Autodesk Inventor part; units mm, degrees
ref_plane "YZ Plane" through (0, 0, 0) normal (1, 0, 0) x (0, 1, 0)
ref_plane "XZ Plane" through (0, 0, 0) normal (0, 1, 0) x (-1, 0, 0)
ref_plane "XY Plane" through (0, 0, 0) normal (0, 0, 1) x (1, 0, 0)
sketch "Sketch1" plane through (0, 0, 0) normal (0, 0, 1) x (1, 0, 0)
  circle A0 centre (0, 0) radius 1.5
  circle A1 centre (0, 0) radius 3
  line L0 (0, 3) -> (28, 3)
  line L1 (28, 3) -> (28, -3)
  line L2 (28, -3) -> (0, -3)
  line L3 (0, -3) -> (0, 3)
  line L4 (28, 3) -> (10, 3)
  line L5 (10, 3) -> (10, 59)
  line L6 (10, 59) -> (28, 59)
  line L7 (28, 59) -> (28, 3)
  circle A2 centre (23.5, 28.5) radius 5.5
  circle A3 centre (15.9973, 49.5) radius 6.25
  line L8 (23.5, 28.5) -> (15.9973, 49.5) construction
  line L9 (23.5, 28.5) -> (10, 28.5) construction
  circle A4 centre (15.9973, 41) radius 1.05
  circle A5 centre (23.3585, 53.75) radius 1.05
  circle A6 centre (8.6361, 53.75) radius 1.05
  line L10 (10, 59) -> (6, 59)
  line L11 (6, 59) -> (6, 45)
  line L12 (6, 45) -> (10, 45)
  line L13 (10, 45) -> (10, 59)
  line L14 (6, 45) -> (10, 41)
  line L15 (6, 45) -> (11.6569, 45) construction
  line L16 (28, 34.5) -> (31, 34.5)
  line L17 (31, 34.5) -> (31, 22.5)
  line L18 (31, 22.5) -> (28, 22.5)
  line L19 (28, 22.5) -> (28, 34.5)
  line L20 (31, 34.5) -> (28, 37.5)
  line L21 (31, 34.5) -> (35.2426, 34.5) construction
  line L22 (31, 22.5) -> (28, 19.5)
  line L23 (31, 22.5) -> (35.2426, 22.5) construction
  circle A7 centre (13.5, 7.5) radius 1.5
  circle A8 centre (17.5, 11.5) radius 1.25
  circle A9 centre (25, 10.5) radius 1.25
  line L24 (15.9973, 49.5) -> (6, 49.5) construction
  line L25 (15.9973, 41) -> (15.9973, 49.5) construction
  circle A10 centre (19.7487, 39) radius 1
  circle A11 centre (15, 29.5) radius 1.05
  circle A12 centre (13, 34) radius 1.05
  circle A13 centre (25, 48) radius 1.05
  line L26 (10, 27) -> (28, 27) construction
  line L27 (28, 27) -> (28, 51) construction
  line L28 (28, 51) -> (10, 51) construction
  line L29 (10, 51) -> (10, 27) construction
  line L30 (11.7876, 31.9) -> (10.5751, 34) construction
  line L31 (10.5751, 34) -> (11.7876, 36.1) construction
  line L32 (11.7876, 36.1) -> (14.2124, 36.1) construction
  line L33 (14.2124, 36.1) -> (15.4249, 34) construction
  line L34 (15.4249, 34) -> (14.2124, 31.9) construction
  line L35 (14.2124, 31.9) -> (11.7876, 31.9) construction
  line L36 (13.7876, 27.4) -> (12.5751, 29.5) construction
  line L37 (12.5751, 29.5) -> (13.7876, 31.6) construction
  line L38 (13.7876, 31.6) -> (16.2124, 31.6) construction
  line L39 (16.2124, 31.6) -> (17.4249, 29.5) construction
  line L40 (17.4249, 29.5) -> (16.2124, 27.4) construction
  line L41 (16.2124, 27.4) -> (13.7876, 27.4) construction
  dimension "d0" = 3
  dimension "d1" = 6
  dimension "d2" = 28
  dimension "d3" = 6
  dimension "d4" = 0
  dimension "d5" = 3
  dimension "d6" = 18
  dimension "d7" = 56
  dimension "d8" = 11
  dimension "d9" = 4.5
  dimension "d10" = 25.5
  dimension "d11" = 12.5
  dimension "d12" = 22.3
  dimension "d14" = 2.1
  dimension "d17" = 9.5
  dimension "d20" = 360
  dimension "d22" = 4
  dimension "d23" = 14
  dimension "d24" = 45
  dimension "d25" = 3
  dimension "d26" = 12
  dimension "d27" = 6
  dimension "d28" = 135
  dimension "d29" = 135
  dimension "d32" = 3
  dimension "d33" = 10.5
  dimension "d34" = 3.5
  dimension "d35" = 2.5
  dimension "d36" = 14.5
  dimension "d37" = 7.5
  dimension "d38" = 2.5
  dimension "d39" = 15
  dimension "d40" = 13.5
  dimension "d60" = 8.5
  dimension "d61" = 270
  dimension "d82" = 2
  dimension "d83" = 11.15
  dimension "d84" = 2.1
  dimension "d85" = 2.1
  dimension "d86" = 2.1
  dimension "d87" = 5
  dimension "d88" = 3
  dimension "d89" = 25
  dimension "d90" = 29.5
  dimension "d91" = 3
  dimension "d92" = 11
  dimension "d93" = 24
  dimension "d94" = 8
  dimension "d101" = 2.1
  dimension "d102" = 2.1
extrude "Extrusion1" add sketch "Sketch1" along normal blind 5 contours A0 L3 A1 | A0 L3 A1 | L0 L1 L2 A1 | L5 A3 L6 L7 A2 L0 | L14 L12 L5 | L7 L18 L22 | L12 L11 L10 L5 A3 | L7 A2 L16 L17 L18 | L16 L7 L20
fillet "Fillet1" radius 2 1 edges at (28, -3, 2.5)
fillet "Fillet2" radius 2 1 edges at (10, 3, 2.5)
sketch "Sketch2" plane through (0, 0, 5) normal (0, 0, 1) x (1, 0, 0)
  line L0 (28, -1) -> (28, 19.5)
  line L1 (0, -3) -> (26, -3)
  line L2 (28, -1) -> (28, 19.5)
  line L3 (28, 20.75) -> (15.25, 20.75)
  line L4 (15.25, 20.75) -> (15.25, 0.75)
  line L5 (15.25, 0.75) -> (28, 0.75)
  line L6 (28, 0.75) -> (28, 20.75)
  line L7 (28, 19.5) -> (31, 22.5)
  line L8 (28, 20.75) -> (29.25, 20.75)
  line L9 (28, 19.5) -> (31, 22.5)
  line L10 (26.75, 20.75) -> (26.75, 0.75)
  point P0 (0, 0)
  point P1 (28, 19.5)
  point P2 (28, 19.5)
  dimension "d43" = 12.75
  dimension "d44" = 20
  dimension "d45" = 23.75
extrude "Extrusion2" cut sketch "Sketch2" against normal blind 3
sketch "Sketch3" plane through (6, 59, 0) normal (0, 1, 0) x (1, 0, 0)
  circle A0 centre (3, -2.5) radius 1
  line L0 (22, 0) -> (0, 0)
  line L1 (0, 0) -> (0, -5)
  line L2 (22, -5) -> (0, -5)
  line L3 (22, 0) -> (22, -5)
  circle A1 centre (19, -2.5) radius 1
  dimension "d48" = 2
  dimension "d49" = 2
  dimension "d50" = 2.5
  dimension "d51" = 2.5
  dimension "d52" = 3
  dimension "d53" = 3
extrude "Extrusion3" cut sketch "Sketch3" against normal blind 3 contours A0 | A1
thread "Thread1"
thread "Thread2"
sketch "Sketch5" plane through (0, 0, 5) normal (0, 0, 1) x (1, 0, 0)
  circle A0 centre (15.9973, 41) radius 1.05
  circle A1 centre (8.6361, 53.75) radius 1.05
  circle A2 centre (23.3585, 53.75) radius 1.05
  circle A3 centre (15.9973, 41) radius 2
  circle A4 centre (8.6361, 53.75) radius 2
  circle A5 centre (23.3585, 53.75) radius 2
  point P0 (0, 0)
  dimension "d62" = 4
  dimension "d63" = 4
  dimension "d64" = 4
extrude "Extrusion4" cut sketch "Sketch5" against normal blind 3 contours A0 | A1 | A2 | A3 | A4 | A5
sketch "Sketch7" plane through (0, 0, 5) normal (0, 0, 1) x (1, 0, 0)
  circle A0 centre (13.5, 7.5) radius 1.5
  circle A1 centre (13.5, 7.5) radius 2.75
  point P0 (0, 0)
  dimension "d67" = 5.5
extrude "Extrusion5" cut sketch "Sketch7" against normal blind 2 contours A0 | A1
sketch "Sketch8" plane through (0, 0, 5) normal (0, 0, 1) x (1, 0, 0)
  line L0 (10, 59) -> (10, 56)
  line L1 (8, 59) -> (8, 56)
  circle A0 centre (23.3585, 53.75) radius 2
  circle A1 centre (8.6361, 53.75) radius 2
  circle A2 centre (15.9973, 41) radius 2
  circle A3 centre (23.5, 28.5) radius 5.5
  circle A4 centre (15.9973, 49.5) radius 6.25
  arc A5 (15.25, 9.6213) -> (15.25, 5.3787) centre (13.5, 7.5) ccw
  line L2 (15.25, 9.6213) -> (15.25, 20.75)
  line L3 (15.25, 20.75) -> (29.25, 20.75)
  line L4 (29.25, 20.75) -> (31, 22.5)
  line L5 (31, 22.5) -> (31, 34.5)
  line L6 (31, 34.5) -> (28, 37.5)
  line L7 (28, 37.5) -> (28, 59)
  line L8 (28, 59) -> (6, 59)
  line L9 (6, 59) -> (6, 45)
  line L10 (6, 45) -> (10, 41)
  line L11 (10, 41) -> (10, 5)
  line L12 (24, 59) -> (24, 56)
  line L13 (26, 59) -> (26, 56)
  line L14 (7, 56.275) -> (11, 56.275)
  line L15 (11, 56.275) -> (11, 58.125)
  line L16 (11, 58.125) -> (7, 58.125)
  line L17 (7, 58.125) -> (7, 56.275)
  line L18 (7, 56.275) -> (11, 58.125) construction
  line L19 (11, 56.275) -> (7, 58.125) construction
  line L20 (23, 58.125) -> (27, 58.125)
  line L21 (27, 58.125) -> (27, 56.275)
  line L22 (27, 56.275) -> (23, 56.275)
  line L23 (23, 56.275) -> (23, 58.125)
  line L24 (23, 58.125) -> (27, 56.275) construction
  line L25 (27, 58.125) -> (23, 56.275) construction
  arc A6 (8, 3) -> (10, 5) centre (8, 5) ccw
  line L26 (8, 3) -> (0, 3)
  arc A7 (0, 3) -> (0, -3) centre (0, 0) ccw
  line L27 (0, -3) -> (26, -3)
  arc A8 (26, -3) -> (28, -1) centre (26, -1) ccw
  line L28 (28, -1) -> (28, 0.75)
  line L29 (28, 0.75) -> (15.25, 0.75)
  line L30 (15.25, 0.75) -> (15.25, 5.3787)
  point P0 (9, 57.2)
  point P1 (25, 57.2)
  dimension "d70" = 4
  dimension "d71" = 1.85
  dimension "d72" = 4
  dimension "d73" = 1.85
  dimension "d74" = 1
  dimension "d75" = 1.8
  dimension "d76" = 1.8
  dimension "d77" = 1
extrude "Extrusion6" cut sketch "Sketch8" against normal up to surface (5 mm away) contours L16 L15 L14 L0 | L0 L14 L1 L16 | L1 L14 L17 L16 | L20 L13 L22 L12 | L12 L22 L23 L20 | L20 L21 L22 L13
sketch "Sketch10" plane through (0, 0, 0) normal (0, 0, -1) x (-1, 0, 0)
  circle A0 centre (-25, 48) radius 1.05
  circle A1 centre (-13, 34) radius 1.05
  circle A2 centre (-15, 29.5) radius 1.05
  line L0 (-26.2124, 45.9) -> (-27.4249, 48)
  line L1 (-27.4249, 48) -> (-26.2124, 50.1)
  line L2 (-26.2124, 50.1) -> (-23.7876, 50.1)
  line L3 (-23.7876, 50.1) -> (-22.5751, 48)
  line L4 (-22.5751, 48) -> (-23.7876, 45.9)
  line L5 (-23.7876, 45.9) -> (-26.2124, 45.9)
  line L6 (-16.2124, 27.4) -> (-17.4249, 29.5)
  line L7 (-17.4249, 29.5) -> (-16.2124, 31.6)
  line L8 (-16.2124, 31.6) -> (-13.7876, 31.6)
  line L9 (-13.7876, 31.6) -> (-12.5751, 29.5)
  line L10 (-12.5751, 29.5) -> (-13.7876, 27.4)
  line L11 (-13.7876, 27.4) -> (-16.2124, 27.4)
  line L12 (-14.2124, 31.9) -> (-15.4249, 34)
  line L13 (-15.4249, 34) -> (-14.2124, 36.1)
  line L14 (-14.2124, 36.1) -> (-11.7876, 36.1)
  line L15 (-11.7876, 36.1) -> (-10.5751, 34)
  line L16 (-10.5751, 34) -> (-11.7876, 31.9)
  line L17 (-11.7876, 31.9) -> (-14.2124, 31.9)
  point P0 (0, 0)
  point P1 (-13.9053, 32.1)
  point P2 (-12.0947, 30.9)
  dimension "d95" = 2.1
  dimension "d96" = 2.1
  dimension "d98" = 2.1
extrude "Extrusion7" cut sketch "Sketch10" against normal blind 1.8 contours A1 | A2 | L0 L1 L2 L3 L4 L5 | L6 L7 L8 L9 L10 L11 | L12 L13 L14 L15 L16 L17
properties part number "PartA_3D"
Source: CAD feature listing. Evaluate the final solid. Frame: model axes, mm. A direction names the side the tool comes from. Coordinates: 2 decimals unless noted, no trailing zeros. Loops run counter-clockwise (first coordinate to the right, second up) from the corner with the lowest first, then second, coordinate; pieces in that order, holes last. Notation, with made-up numbers: (-10, 61) -> (36, 61) arc R22 ccw to (36, 68) -> close; hole circle Ø5 at (10.25, -3). An arc over 180 degrees is marked (long way). One line per item, written item: value. Start each with the question number.
Q1. Set-up query: faces 5 (the face through (16.827, 30.535, 0.887)), 6 (the face through (25, 56, 2)), 7 (the face through (11, 57, 3)). Return all of +Z, -Z, +X, -X, +Y, -Y with unobstructed straight access to the full face (end or side cutting, diameter ignored); none if empty.
Q2. Mould query, pull axis Z, two halves, no side actions, for faces 1 (the face through (25, 58.125, 4)), 2 (the face through (24.22, 52.89, 2)), 3 (the face through (9, 56, 2)), 4 (the face through (8.2, 58.6, 3.1)). Classes: pulls with the +Z half, pulls with the -Z half, needs draft (parallel to the pull), parting line crosses it, or undercut.
Q3. Contact query for flat-ended pins moving along their axis: P1, Ø3, axis at y = 42, z = 1.5, coming from the +X side; P2, Ø7, axis at x = 22.5, y = 7.5, coming from the +Z side; P3, Ø1.5, axis at y = 50, z = 3, coming from the -X side. Output: stop coordinate, or through.
Q4. Line query: line 1 along X through (y, z) = (58.65, 2.5); line 2 along Z through (x, y) = (25, 58.4); line 3 along Y through (x, z) = (20.5, 2.1). Output: solid intervals per line, ascending.
Q5. Section query A-A, the plane y = 0. Return the cut outline in (x, z), and give its area (3 significant figures).
Q6. Section query B-B, the plane x = 9. Return the cut outline in (y, z) (3 decimals).
Results:
1. face 5: -Z
1. face 6: +Y
1. face 7: +Z, -Z
2. face 1: needs draft
2. face 2: pulls with the +Z half
2. face 3: undercut
2. face 4: undercut
3. P1: x = 28
3. P2: z = 2
3. P3: x = 6
4. line 1: 6 to 8, 10 to 24, 26 to 28
4. line 2: 0 to 1.5, 3.5 to 5
4. line 3: -3 to 0.75, 20.75 to 23.89, 33.11 to 38.34, 39.66 to 45.17, 53.83 to 59
5. outline: (-3, 0) -> (-1.5, 0) -> (-1.5, 5) -> (-3, 5) -> close; (1.5, 0) -> (28, 0) -> (28, 5) -> (1.5, 5) -> close
5. area: 140 mm^2
6. outline: (-3, 0) -> (3.268, 0) -> (3.268, 5) -> (-3, 5) -> close; (42, 0) -> (52.765, 0) -> (52.765, 2) -> (51.783, 2) -> (51.783, 5) -> (42, 5) -> close; (54.735, 0) -> (56.275, 0) -> (56.275, 1.5) -> (56, 1.5) -> (56, 3.5) -> (56.275, 3.5) -> (56.275, 5) -> (55.717, 5) -> (55.717, 2) -> (54.735, 2) -> close; (58.125, 0) -> (59, 0) -> (59, 1.5) -> (58.125, 1.5) -> close; (58.125, 3.5) -> (59, 3.5) -> (59, 5) -> (58.125, 5) -> close
